The model under review builds one solid part; all positions refer to its coordinate system, in mm. Coordinates: 2 decimals unless noted, no trailing zeros. Write each loop counter-clockwise with the first axis right and the second up, starting at its lowest first coordinate (ties: lowest second). Pieces come first, ordered by that corner, then holes. Notation, with made-up numbers: (-37.75, 27.5) -> (-15.75, 27.5) arc R28 ccw to (-15.75, 52.5) -> close; hole circle Ø4 at (-13.5, 81.25). An arc over 180 degrees is marked (long way). Put each result on its own line as item: value. Start each with the question number.
Autodesk Inventor part; units mm, degrees
ref_plane "YZ Plane" through (0, 0, 0) normal (1, 0, 0) x (0, 1, 0)
ref_plane "XZ Plane" through (0, 0, 0) normal (0, 1, 0) x (-1, 0, 0)
ref_plane "XY Plane" through (0, 0, 0) normal (0, 0, 1) x (1, 0, 0)
sketch "Boceto1" plane through (0, 0, 0) normal (0, 1, 0) x (-1, 0, 0)
  circle A0 centre (0, 0) radius 8
  dimension "d0" = 16
extrude "Extrusión1" add sketch "Boceto1" along normal blind 9.1
sketch "Boceto2" plane through (0, 9.1, 0) normal (0, 1, 0) x (1, 0, 0)
  circle A0 centre (0, 0) radius 2.65
  dimension "d3" = 5.3
extrude "Extrusión2" cut sketch "Boceto2" against normal through all
sketch "Boceto3" plane through (0, 9.1, 0) normal (0, 1, 0) x (1, 0, 0)
  circle A0 centre (0, 0) radius 3.85
  circle A1 centre (0, 0) radius 2.65
  dimension "d6" = 7.7
extrude "Extrusión3" add sketch "Boceto3" along normal blind 7
sketch "Boceto4" plane through (0, 0, 0) normal (0, -1, 0) x (1, 0, 0)
  circle A0 centre (0, 0) radius 10
  dimension "d9" = 20
extrude "Extrusión4" add sketch "Boceto4" against normal blind 2
chamfer "Chaflán1" distance 7 angle 15 1 edges at (8, 2, 0) measured on face at (-7.8964, 4.3667, 1.2833)
sketch "Boceto5" plane through (0, 2, 0) normal (0, 1, 0) x (1, 0, 0)
  circle A0 centre (0, 0) radius 2.65
extrude "Extrusión5" cut sketch "Boceto5" against normal through all
properties part number "elbowsupport"
1. Consider section D-D on y = 1.5. State the section outline as (x, z) points, then the cut area to 3 significant figures.
2. Consider section C-C on y = 12.75. State the section outline as (x, z) points.
3. Insertion check: P1, Ø3, axis at x = -3, y = 13, coming from the -Z side; P2, Ø8, axis at y = 13.5, z = 5, coming from the -X side; P3, Ø3, axis at x = 0.5, y = 4, coming from the -Z side; P4, Ø5, axis at x = 2, z = -1, coming from the +Y side. Each pin has a flat end and moves straight along its axis. Give the tip position at first contact, or say it passes through.
4. Consider section B-B on z = 0. State the section outline as (x, y) points, then the cut area to 3 significant figures.
5. Wall thickness on line 1 (Z direction, x = 0, y = 12.5); line 2 (X direction, y = 9, z = 0): over which ranges is each line inside the solid? List them lowest first. Write a range as from..to.
6. Consider section A-A on x = 0. State the section outline as (y, z) points, then the cut area to 3 significant figures.
7. The part is to be moulded in two halves that separate along Z. For faces 1 (the flat face through (-2, 9.1, 4)), 2 (the cylindrical face through (-0.83, 12.55, -3.76)), 3 (the cylindrical face through (2.45, 7.94, -1.01)), say which applies: released by +Z, released by -Z, zero draft, split by the parting line, or undercut.
Output values:
1. outline: circle Ø20 at (0, 0); hole circle Ø5.3 at (0, 0)
1. area: 292 mm^2
2. outline: circle Ø7.7 at (0, 0); hole circle Ø5.3 at (0, 0)
3. P1: stops at z = -3.55
3. P2: stops at x = -3.72
3. P3: stops at z = -9.73
3. P4: stops at y = 16.1
4. outline: (-10, 0) -> (-2.65, 0) -> (-2.65, 16.1) -> (-3.85, 16.1) -> (-3.85, 9.1) -> (-8, 9.1) -> (-8, 9) -> (-9.88, 2) -> (-10, 2) -> close; (2.65, 0) -> (10, 0) -> (10, 2) -> (9.88, 2) -> (8, 9) -> (8, 9.1) -> (3.85, 9.1) -> (3.85, 16.1) -> (2.65, 16.1) -> close
4. area: 135 mm^2
5. line 1: z = -3.85..-2.65, 2.65..3.85
5. line 2: x = -8..-2.65, 2.65..8
6. outline: (0, -10) -> (2, -10) -> (2, -9.88) -> (9, -8) -> (9.1, -8) -> (9.1, -3.85) -> (16.1, -3.85) -> (16.1, -2.65) -> (0, -2.65) -> close; (0, 2.65) -> (16.1, 2.65) -> (16.1, 3.85) -> (9.1, 3.85) -> (9.1, 8) -> (9, 8) -> (2, 9.88) -> (2, 10) -> (0, 10) -> close
6. area: 135 mm^2
7. face 1: zero draft
7. face 2: split by the parting line
7. face 3: undercut
